```python
from build123d import *

# Parameters (mm, degrees)
F0_W          = 150
F0_H          = 200
F1_DEPTH      = 3
F1_DEPTH_BACK = 3
F2_R          = 10
F4_D          = 3
F4_DEPTH      = 12
F5_W          = 16
F5_H          = 20
F5_R          = 1.5
F5_R_2        = 5
F5_R_3        = 3
F6_DEPTH      = 25


with BuildPart() as f1:
    # F0 (on Front) → F1 (new body, two sides)
    with BuildSketch(Plane.XZ) as f1_sk:
        Rectangle(F0_W, F0_H)
    extrude(amount=F1_DEPTH)
    extrude(f1_sk.sketch, amount=-F1_DEPTH_BACK)

    # F2
    f2_edges = [f1.edges().sort_by_distance(p)[0] for p in [
        (-75, 0, -100),
        (75, 0, -100),
        (75, 0, 100),
        (-75, 0, 100),
    ]]
    fillet(f2_edges, radius=F2_R)

    # F4
    with Locations(Plane.XZ.offset(3)):
        with Locations((62.5, -80), (62.5, -50), (62.5, 50), (62.5, 80), (-62.5, 80), (-62.5, 50), (-62.5, -50), (-62.5, -80)):
            Hole(F4_D / 2, depth=F4_DEPTH)

    # F5 (on face) → F6 (cut)
    with BuildSketch(Plane.XZ.offset(3)):
        with Locations((-40, 0)):
            Rectangle(F5_W, F5_H)
        with BuildLine():
            ThreePointArc((12.5, 21), (14, 22.5), (12.5, 24))
            Line((12.5, 24), (-12.5, 24))
            ThreePointArc((-12.5, 24), (-14, 22.5), (-12.5, 21))
            Line((-12.5, 21), (12.5, 21))
        make_face()
        with BuildLine():
            ThreePointArc((12.5, -24), (14, -22.5), (12.5, -21))
            Line((12.5, -21), (-12.5, -21))
            ThreePointArc((-12.5, -21), (-14, -22.5), (-12.5, -24))
            Line((-12.5, -24), (12.5, -24))
        make_face()
        with Locations((40, 0)):
            Rectangle(F5_W, F5_H)
        with Locations((20, 0)):
            Circle(F5_R)
        with Locations((0, -65)):
            Circle(F5_R_2)
        with Locations((-38.842574, -47.822315)):
            Circle(F5_R_3)
        with Locations((38.842574, -47.822315)):
            Circle(F5_R_3)
        with Locations((0, -90)):
            Circle(F5_R_3)
        with Locations((-20, 0)):
            Circle(F5_R)
        with Locations((15, -90)):
            Circle(F5_R)
        with Locations((-15, -90)):
            Circle(F5_R)
        with Locations((0, 65)):
            Circle(F5_R_2)
        with Locations((0, 90)):
            Circle(F5_R_3)
        with Locations((-15, 90)):
            Circle(F5_R)
        with Locations((15, 90)):
            Circle(F5_R)
    extrude(amount=-F6_DEPTH, mode=Mode.SUBTRACT)


solid = f1.part
```
For this review, take the finished solid that the model builds, in its own axes (mm). A direction names the side the tool comes from. Coordinates: 2 decimals unless noted, no trailing zeros. Loops run counter-clockwise (first coordinate to the right, second up) from the corner with the lowest first, then second, coordinate; pieces in that order, holes last. Notation, with made-up numbers: (-32.5, 26.5) - (-12.5, 26.5) arc R26 cw to (-12.5, 49.5) - close; hole circle Ø2 at (-19, 7.5). An arc over 180 degrees is marked (long way). Use one line per item in the form item = value. Start each with the question number.
1) Take a section at A-A (z = 65). State the section outline as (x, y) points.
2) Draft analysis for pull direction X (two halves, no side actions). For faces 3 (the face through (-1, 3, 1)), 4 (the face through (41.704, -0.042, -46.921)), 5 (the face through (-75, 0, -1)), 6 (the face through (0, 0, -21)), state which applies: released by +X, released by -X, zero draft, split by the parting line, or undercut.
3) Take a section at C-C (y = -1.3). State how many separate pieces and enclosed holes the cut face has, plus the area to 3 significant figures.
4) Take a section at B-B (z = -6.5). State the section outline as (x, y) points.
5) For pin 1 (2.5 mm diameter, centred on x = -62.5, z = 50, fed in from +Y), flat-tipped, find the tip position at first contact; note if it passes through.
6) To check wall thickness, follow probe 1 along X at (y, z) = (-0.6, 80); probe 2 along Z at (x, y) = (-9, 1.7); probe 3 along X at (y, z) = (-1.9, -4). State the ranges of each line that lie inside material, in increasing order. Write a range as from..to.
7) For faces 1 (the face through (-1, 0, 100)), 2 (the face through (-48, 0, 0)), list the 3-axis set-ups (+Z, -Z, +X, -X, +Y, -Y) from which the entire face can be reached by the end or side of a thin tool; tool diameter is ignored.
From the geometry:
q1.outline = (-75, -3) - (-5, -3) - (-5, 3) - (-75, 3) - close; (5, -3) - (75, -3) - (75, 3) - (5, 3) - close
q2.face_3 = zero draft
q2.face_4 = undercut
q2.face_5 = released by -X
q2.face_6 = undercut
q3.separate_pieces = 1
q3.enclosed_holes = 24
q3.area = 28,700 mm2
q4.outline = (-75, -3) - (-48, -3) - (-48, 3) - (-75, 3) - close; (-32, -3) - (32, -3) - (32, 3) - (-32, 3) - close; (48, -3) - (75, -3) - (75, 3) - (48, 3) - close
q5.pin_1 = through
q6.probe_1 = -75..-64, -61..61, 64..75
q6.probe_2 = -100..-24, -21..21, 24..100
q6.probe_3 = -75..-48, -32..32, 48..75
q7.face_1 = +Z, +X, -X, +Y, -Y
q7.face_2 = +Y, -Y
